```python
from build123d import *

# Parameters (mm, degrees)
F1_DEPTH = 127
F2_W     = 68.072
F2_H     = 13.462
F3_DEPTH = 13.462
F5_DEPTH = 12.7


with BuildPart() as f1:
    # F0 (on Right) → F1 (new body)
    with BuildSketch(Plane.YZ):
        Polygon((60.512159, 34.029547), (-66.487841, 0), (60.512159, 0), align=None)
    extrude(amount=F1_DEPTH)

    # F2 (on face) → F3 (cut)
    with BuildSketch(Plane(origin=(0, 0, 0), x_dir=(0, -1, 0), z_dir=(-1, 0, 0))):
        with Locations((-23.936159, 6.731)):
            Rectangle(F2_W, F2_H)
    extrude(amount=-F3_DEPTH, mode=Mode.SUBTRACT)

    # F4 (on face) → F5 (cut)
    with BuildSketch(Plane(origin=(0, 60.512159, 0), x_dir=(-1, 0, 0), z_dir=(0, 1, 0))):
        with BuildLine():
            ThreePointArc((-101.6, 23.364774), (-107.95, 17.014774), (-101.6, 10.664774))
            Line((-101.6, 10.664774), (-25.4, 10.664774))
            ThreePointArc((-25.4, 10.664774), (-19.05, 17.014774), (-25.4, 23.364774))
            Line((-25.4, 23.364774), (-101.6, 23.364774))
        make_face()
    extrude(amount=-F5_DEPTH, mode=Mode.SUBTRACT)


solid = f1.part
```
For this review, take the finished solid that the model builds, in its own axes (mm). A direction names the side the tool comes from. Give positions to 0.01 mm unless a question says otherwise; leave off trailing zeros. Order: outer loops, then holes, each group sorted by start corner. A loop starts at its lowest first (then second) coordinate and runs counter-clockwise, first axis right, second up.
1) Take a section at A-A (x = 54.5). Give the boundary of the cut face in (y, z), then the cut area to 3 significant figures.
2) Take a section at C-C (z = 16). Give the boundary of the cut face in (x, y), then the cut area to 3 significant figures.
3) Take a section at D-D (x = 112). Give the boundary of the cut face in (y, z).
4) For faces 5 (the face through (63, 60.512, 9)), 6 (the face through (63, 54, 23.365)), 7 (the face through (7, 24, 13.462)), list the 3-axis set-ups (+Z, -Z, +X, -X, +Y, -Y) from which the entire face can be reached by the end or side of a thin tool; tool diameter is ignored.
5) Wall thickness on line 1 (X direction, y = 20, z = 4.5); line 2 (Z direction, x = 104.5, y = 52); line 3 (Z direction, x = 108, y = -45.5): over which ranges is each line inside the solid? List them lowest first.
6) Take a section at B-B (y = 20.5). Give the boundary of the cut face in (x, z).
7) Insertion check: pin 1 (10 mm diameter, centred on x = 80.5, y = -45, fed in from +Z); pin 2 (14 mm diameter, centred on x = 71, y = 55, fed in from +Z); pin 3 (3 mm diameter, centred on x = 16, y = -20, fed in from +Z). Each pin has a flat end and moves straight along its axis. Give the tip position at first contact, or say it passes through.
8) The part is to be moulded in two halves that separate along X. For faces 1 (the face through (64, 54, 10.665)), 2 (the face through (13.462, 24, 7)), 3 (the face through (64, 47.812, 17)), 4 (the face through (63, -4, 0)), say which applies: released by +X, released by -X, zero draft, split by the parting line, or undercut.
Derived:
1. outline: (-66.49, 0) - (60.51, 0) - (60.51, 10.66) - (47.81, 10.66) - (47.81, 23.36) - (60.51, 23.36) - (60.51, 34.03) - close
1. area: 2,000 mm2
2. outline: (0, -6.78) - (127, -6.78) - (127, 60.51) - (107.87, 60.51) - (107.87, 47.81) - (19.13, 47.81) - (19.13, 60.51) - (0, 60.51) - close
2. area: 7,420 mm2
3. outline: (-66.49, 0) - (60.51, 0) - (60.51, 34.03) - close
4. face 5: +Z, -Z, +X, -X, +Y
4. face 6: +Y
4. face 7: -Z, -X
5. line 1: x = 13.46 to 127
5. line 2: z = 0 to 11.37, 22.66 to 31.75
5. line 3: z = 0 to 5.62
6. outline: (0, 13.46) - (13.46, 13.46) - (13.46, 0) - (127, 0) - (127, 23.31) - (0, 23.31) - close
7. pin 1: stops at z = 7.1
7. pin 2: stops at z = 34.03
7. pin 3: stops at z = 12.86
8. face 1: undercut
8. face 2: released by -X
8. face 3: undercut
8. face 4: zero draft
